Part print with two shaded views. Sizes in mm from the minimum x, y, z corner. A direction names the side the tool comes from. Give positions to 0.01 mm unless a question says otherwise; leave off trailing zeros. Write each loop counter-clockwise with the first axis right and the second up, starting at its lowest first coordinate (ties: lowest second). Pieces come first, ordered by that corner, then holes.
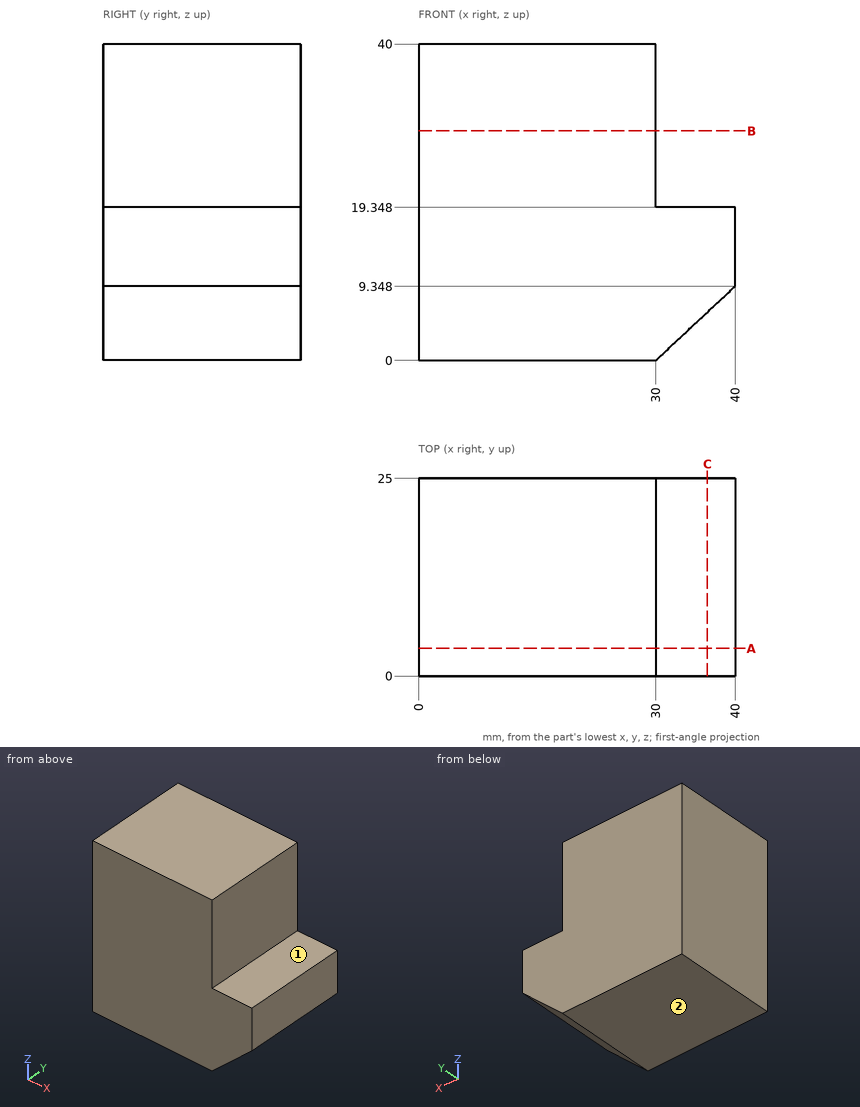
1) Saw through at A-A (y = 3.5). Write the cut outline in (x, z).
Check result:
outline: (0, 0) - (30, 0) - (40, 9.35) - (40, 19.35) - (30, 19.35) - (30, 40) - (0, 40) - close
2) Saw through at B-B (z = 29). Write the cut outline in (x, y).
Check result:
outline: (0, 0) - (30, 0) - (30, 25) - (0, 25) - close
3) 3-axis set-ups, long thin cutter, end or side, ignore diameter. For the marked faces 1 and 2: which of +Z, -Z, +X, -X, +Y, -Y reach the whole face in a straight line?
Check result:
face 1: +Z, +X, +Y, -Y
face 2: -Z, +X, -X, +Y, -Y
4) Drill centre lines: L1, parallel to X at y = 19, z = 25; L2, parallel to Z at x = 35, y = 22.5; L3, parallel to X at y = 14, z = 9. Where is each one in solid material? Low to high.
Check result:
L1: x = 0 to 30
L2: z = 4.67 to 19.35
L3: x = 0 to 39.63
5) Flat gauge pin, fed straight in: P1, Ø11, axis at x = 36, y = 17, coming from the +Z side. Where does the tip first touch, or does it go through?
Check result:
P1: stops at z = 19.35
6) Saw through at C-C (x = 36.5). Write the cut outline in (y, z).
Check result:
outline: (0, 6.08) - (25, 6.08) - (25, 19.35) - (0, 19.35) - close
